The listing builds one solid part. Answer for the finished solid, in the listing's coordinates (mm). A direction names the side the tool comes from. Round coordinates to 2 decimals unless told otherwise and drop trailing zeros. Order: outer loops, then holes, each group sorted by start corner. A loop starts at its lowest first (then second) coordinate and runs counter-clockwise, first axis right, second up. Notation, with made-up numbers: (18.5, 15) - (38.5, 15) arc R21 ccw to (38.5, 33) - close; hole circle Ø4 at (51.25, 63). An arc over 180 degrees is marked (long way). One line per item, written item: value. Start each with the question number.
1. Section A-A, the plane x = 0 is taken. Give the vertices of the cut face in (y, z).
2. For a pull along Y with two mould halves and no side action, classify faces 5 (the flat face through (3, -3, 0)), 6 (the flat face through (-15, 0, 2)), 7 (the flat face through (-10.98, 6.7, -1.23)) as released by +Y, released by -Y, zero draft, split by the parting line, or undercut.
3. Straight lines are drawn through the part: line 1 (Y direction, x = 0, z = 3.85); line 2 (Y direction, x = 14.5, z = 2.5); line 3 (X direction, y = -6, z = 3.75). For each, find the intervals that lie inside material, in ascending order.
4. Section D-D, the plane x = 15.5 is taken. Give the vertices of the cut face in (y, z), then the cut area to 3 significant figures.
5. Section C-C, the plane y = 10 is taken. Give the vertices of the cut face in (x, z), then the cut area to 3 significant figures.
6. Flat-ended cylindrical pins translate along their axes: P1, Ø1.5, axis at x = 10.5, z = 3.5, coming from the +Y side; P2, Ø9, axis at x = 0, y = 0, coming from the -Z side; P3, Ø1.5, axis at y = -1.5, z = 1.5, coming from the -X side. Find the tip coordinate at first contact, or state that the pin passes through.
7. A tool of negligible diameter and unlimited length cuts with its end or side. For faces 1 (the cylindrical face through (17, 5, 1)), 2 (the flat face through (-5.983, 1.77, -1.232)), 3 (the flat face through (-7.45, 5.33, -1.23)), 4 (the cylindrical face through (9.385, 17.465, 1.749)), from which of +Z, -Z, +X, -X, +Y, -Y can it reach the whole face along a straight path? Write none if from no direction.
from build123d import *

# Parameters (mm, degrees)
ESQUISSE2_W              = 30
ESQUISSE2_H              = 30
BOSS_EXTRU_1_DEPTH       = 5
ESQUISSE16_R             = 2.5
BOSS_EXTRU_7_DEPTH       = 6
CONG_3_R                 = 1
ESQUISSE18_R             = 2.5
BOSS_EXTRU_9_DEPTH       = 6
CONG_5_R                 = 1
ESQUISSE8_R              = 12.5
ENL_V_MAT_EXTRU_1_DEPTH  = 2
ESQUISSE19_R             = 7.5
BOSS_EXTRU_10_DEPTH      = 2
ESQUISSE33_R             = 4
ENL_V_MAT_EXTRU_3_DEPTH  = 6
ESQUISSE35_R             = 2.5
BOSS_EXTRU_26_DEPTH      = 6
CONG_6_R                 = 1
BOSS_EXTRU_27_DEPTH      = 2
BOSS_EXTRU_27_DEPTH_BACK = 5.5


with BuildPart() as part:
    # Esquisse2 → Boss.-Extru.1 (new body)
    with BuildSketch(Plane.XY):
        Rectangle(ESQUISSE2_W, ESQUISSE2_H)
    extrude(amount=BOSS_EXTRU_1_DEPTH)

    # Esquisse16 → Boss.-Extru.7 (add)
    with BuildSketch(Plane.ZY.offset(15)):
        with Locations((2.5, 7)):
            Circle(ESQUISSE16_R)
        with Locations((2.5, -7)):
            Circle(ESQUISSE16_R)
    extrude(amount=BOSS_EXTRU_7_DEPTH)

    # Congé3
    cong_3_edges = [part.edges().sort_by_distance(p)[0] for p in [
        (-21, 7, 0),
        (-21, -7, 0),
    ]]
    fillet(cong_3_edges, radius=CONG_3_R)

    # Esquisse18 → Boss.-Extru.9 (add)
    with BuildSketch(Plane(origin=(15, 0, 0), x_dir=(0, 0, -1), z_dir=(1, 0, 0))):
        with Locations((-2.5, 7)):
            Circle(ESQUISSE18_R)
    extrude(amount=BOSS_EXTRU_9_DEPTH)

    # Congé5
    cong_5_edges = [part.edges().sort_by_distance(p)[0] for p in [
        (21, 7, 5),
    ]]
    fillet(cong_5_edges, radius=CONG_5_R)

    # Esquisse8 → Enlèv. mat.-Extru.1 (cut)
    with BuildSketch(Plane.XY.offset(5)):
        Circle(ESQUISSE8_R)
    extrude(amount=-ENL_V_MAT_EXTRU_1_DEPTH, mode=Mode.SUBTRACT)

    # Esquisse19 → Boss.-Extru.10 (add)
    with BuildSketch(Plane.XY.offset(3)):
        Circle(ESQUISSE19_R)
    extrude(amount=BOSS_EXTRU_10_DEPTH)

    # Esquisse33 → Enlèv. mat.-Extru.3 (cut, through all)
    with BuildSketch(Plane.XY.offset(5)):
        Circle(ESQUISSE33_R)
    extrude(amount=-ENL_V_MAT_EXTRU_3_DEPTH, mode=Mode.SUBTRACT)

    # Esquisse35 → Boss.-Extru.26 (add)
    with BuildSketch(Plane(origin=(0, 15, 0), x_dir=(1, 0, 0), z_dir=(0, 1, 0))):
        with Locations((7, -2.5)):
            Circle(ESQUISSE35_R)
    extrude(amount=BOSS_EXTRU_26_DEPTH)

    # Congé6
    cong_6_edges = [part.edges().sort_by_distance(p)[0] for p in [
        (4.5, 21, 2.5),
    ]]
    fillet(cong_6_edges, radius=CONG_6_R)

    # Esquisse31 → Boss.-Extru.27 (add, two sides)
    with BuildSketch(Plane.XY.offset(3)) as boss_extru_27_sk:
        Polygon((-12.02081528, 5.656854249), (-9.899494937, 7.778174593), (-4.937341349, 2.816021005), (-7.058661692, 0.694700662), align=None)
    extrude(amount=BOSS_EXTRU_27_DEPTH)
    extrude(boss_extru_27_sk.sketch, amount=-BOSS_EXTRU_27_DEPTH_BACK)


solid = part.part
Answer list:
1. outline: (-15, 0) - (-4, 0) - (-4, 5) - (-7.5, 5) - (-7.5, 3) - (-12.5, 3) - (-12.5, 5) - (-15, 5) - close; (4, 0) - (15, 0) - (15, 5) - (12.5, 5) - (12.5, 3) - (7.5, 3) - (7.5, 5) - (4, 5) - close
2. face 5: zero draft
2. face 6: undercut
2. face 7: released by +Y
3. line 1: y = -15 to -12.5, -7.5 to -4, 4 to 7.5, 12.5 to 15
3. line 2: y = -15 to 15
3. line 3: x = -20.99 to -10.97, -4.5 to 4.5, 10.97 to 15
4. outline: circle Ø5 at (7, 2.5)
4. area: 19.6 mm²
5. outline: (-15, 0) - (15, 0) - (15, 5) - (7.5, 5) - (7.5, 3) - (-7.5, 3) - (-7.5, 5) - (-15, 5) - close
5. area: 120 mm²
6. P1: stops at y = 15
6. P2: stops at z = 0
6. P3: stops at x = -15
7. face 1: +X
7. face 2: -Z, +X, -Y
7. face 3: -Z, +X, +Y
7. face 4: +Y
